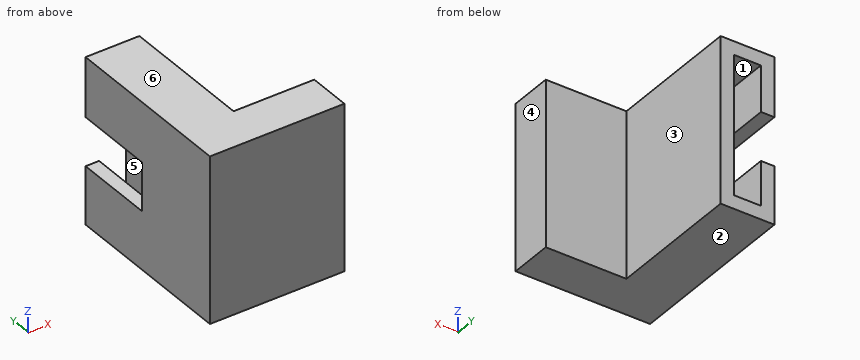
Autodesk Inventor part; units mm, degrees
ref_plane "YZ Plane" through (0, 0, 0) normal (1, 0, 0) x (0, 1, 0)
ref_plane "XZ Plane" through (0, 0, 0) normal (0, 1, 0) x (-1, 0, 0)
ref_plane "XY Plane" through (0, 0, 0) normal (0, 0, 1) x (1, 0, 0)
sketch "Sketch1" plane through (0, 0, 0) normal (0, 1, 0) x (-1, 0, 0)
  line L0 (0, 0) -> (5, 0)
  line L1 (5, 0) -> (5, -25.8)
  line L2 (5, -25.8) -> (0, -25.8)
  line L3 (0, -25.8) -> (0, 0)
  line L4 (7.5, -28.3) -> (7.5, 2.5)
  line L5 (7.5, 2.5) -> (-2.5, 2.5)
  line L6 (-2.5, 2.5) -> (-2.5, -28.3)
  line L7 (-2.5, -28.3) -> (7.5, -28.3)
  dimension "d0" = 5
  dimension "d1" = 25.8
  dimension "d2" = 2.5
extrude "Extrusion1" add sketch "Sketch1" along normal blind 25
sketch "Sketch2" plane through (0, 0, 0) normal (0, -1, 0) x (1, 0, 0)
  line L0 (2.5, -28.3) -> (-7.5, -28.3)
  line L1 (-7.5, 2.5) -> (2.5, 2.5)
  line L2 (2.5, -28.3) -> (-7.5, -28.3)
  line L3 (-7.5, -28.3) -> (-7.5, 2.5)
  line L4 (-7.5, 2.5) -> (2.5, 2.5)
  line L5 (2.5, 2.5) -> (2.5, -28.3)
  point P0 (0, 0)
  point P1 (2.5, 2.5)
extrude "Extrusion2" add sketch "Sketch2" along normal blind 8
sketch "Sketch3" plane through (2.5, 25, 2.5) normal (1, 0, 0) x (0, 0, -1)
  line L0 (30.8, -33) -> (0, -33)
  line L1 (0, -33) -> (0, 0)
  line L2 (30.8, -33) -> (0, -33)
  line L3 (0, -33) -> (0, -25)
  line L4 (0, -25) -> (30.8, -25)
  line L5 (30.8, -25) -> (30.8, -33)
  point P0 (2.5, -25)
  dimension "d7" = 8
extrude "Extrusion3" add sketch "Sketch3" along normal blind 15
sketch "Sketch4" plane through (0, 25, 0) normal (0, 1, 0) x (1, 0, 0)
  line L0 (-5, 0) -> (-5, 25.8)
  line L1 (-7.5, -2.5) -> (-7.5, 28.3)
  line L2 (-5, 17.55) -> (-7.5, 17.55)
  line L3 (-7.5, 17.55) -> (-7.5, 8.55)
  line L4 (-7.5, 8.55) -> (-5, 8.55)
  line L5 (-5, 8.55) -> (-5, 17.55)
  line L6 (2.5, 28.3) -> (-7.5, 28.3)
  point P0 (0, 0)
  point P1 (-5, 8.55)
  point P2 (-7.5, 17.55)
  dimension "d10" = 9
  dimension "d11" = 10.75
extrude "Extrusion4" cut sketch "Sketch4" against normal blind 15
properties part number "base camera"
The model under review builds one solid part; all positions refer to its coordinate system, in mm. Face numbers are marked on the shaded views. A direction names the side the tool comes from. Give positions to 0.01 mm unless a question says otherwise; leave off trailing zeros. Write each loop counter-clockwise with the first axis right and the second up, starting at its lowest first coordinate (ties: lowest second). Pieces come first, ordered by that corner, then holes. Notation, with made-up numbers: (5.5, 25) - (40.5, 25) arc R17 cw to (40.5, 30) - close; hole circle Ø9 at (63.25, 62.5). An arc over 180 degrees is marked (long way). Answer in a Markdown table with one row per item. Add a question column.
1. Tool access review of the marked faces 1, 2 and 3: name each direction out of +Z, -Z, +X, -X, +Y, -Y from which nothing blocks a thin tool from reaching the whole face with its end or side.
2. Wall thickness on line 1 along X through (y, z) = (22, -19); line 2 along Z through (x, y) = (-6, 19.5); line 3 along Z through (x, y) = (-2.5, 20): over which ranges is each line inside the solid? List them lowest first. Write a range as [from, to].
3. We need section A-A on y = 9.5. Write out the cut boundary in (x, z), then the cut area to 3 significant figures.
4. Insertion check: P1, Ø1.5, axis at x = -1.5, z = -8.5, coming from the +Y side; P2, Ø3, axis at x = -6.5, z = -14, coming from the +Y side; P3, Ø3, axis at x = 8.5, y = 3, coming from the +Z side; P4, Ø3, axis at y = 12, z = -6, coming from the +X side. Each pin has a flat end and moves straight along its axis. Give the tip position at first contact, or say it passes through.
5. We need section C-C on z = -18.5. Write out the cut boundary in (x, y), then the cut area to 3 significant figures.
6. We need section B-B on x = -2. Write out the cut boundary in (y, z), then the cut area to 3 significant figures.
7. We need section D-D on y = 13.5. Write out the cut boundary in (x, z).
8. Draft analysis for pull direction Z (two halves, no side actions). For the marked faces 4, 5 and 6, state which applies: +Z half, -Z half, draft (parallel to the pull), parting line (faces both ways), or undercut.
Ans:
| question | item | result |
|---|---|---|
| 1 | face 1 | +Y |
| 1 | face 2 | -Z, +X, -X, +Y, -Y |
| 1 | face 3 | +Z, -Z, +X, +Y |
| 2 | line 1 | x = [-7.5, -5], [0, 2.5] |
| 2 | line 2 | z = [-28.3, -17.55], [-8.55, 2.5] |
| 2 | line 3 | z = [-28.3, -25.8], [0, 2.5] |
| 3 | outline | (-7.5, -28.3) - (2.5, -28.3) - (2.5, 2.5) - (-7.5, 2.5) - close; hole (-5, -25.8) - (0, -25.8) - (0, 0) - (-5, 0) - close |
| 3 | area | 179 mm^2 |
| 4 | P1 | stops at y = 0 |
| 4 | P2 | stops at y = 10 |
| 4 | P3 | passes through |
| 4 | P4 | stops at x = 2.5 |
| 5 | outline | (-7.5, -8) - (17.5, -8) - (17.5, 0) - (2.5, 0) - (2.5, 25) - (0, 25) - (0, 0) - (-5, 0) - (-5, 25) - (-7.5, 25) - close |
| 5 | area | 325 mm^2 |
| 6 | outline | (-8, -28.3) - (25, -28.3) - (25, -25.8) - (0, -25.8) - (0, 0) - (25, 0) - (25, 2.5) - (-8, 2.5) - close |
| 6 | area | 371 mm^2 |
| 7 | outline | (-7.5, -28.3) - (2.5, -28.3) - (2.5, 2.5) - (-7.5, 2.5) - (-7.5, -8.55) - (-5, -8.55) - (-5, 0) - (0, 0) - (0, -25.8) - (-5, -25.8) - (-5, -17.55) - (-7.5, -17.55) - close |
| 8 | face 4 | draft |
| 8 | face 5 | undercut |
| 8 | face 6 | +Z half |
